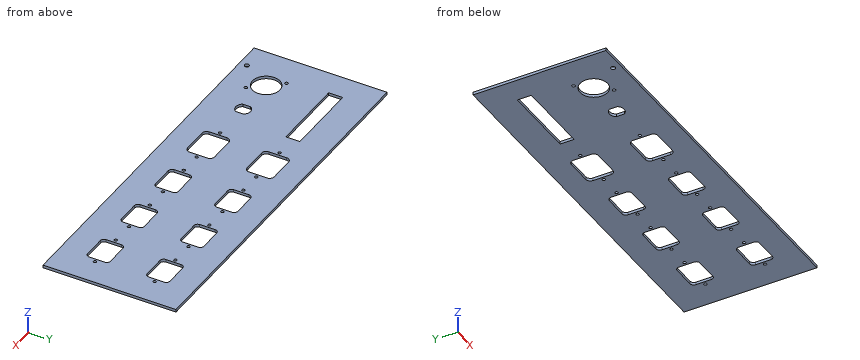
from build123d import *

# Parameters (mm, degrees)
F0_W     = 404
F0_H     = 145
F2_DEPTH = 3
F3_D     = 3.3
F3_DEPTH = 8.6
F3_TIP   = 0.9914200214
F1_R     = 1.5
F1_R_2   = 15
F1_R_3   = 1.75
F1_W     = 82
F1_H     = 15.3
F1_R_4   = 2.5
F4_DEPTH = 25


with BuildPart() as f2:
    # F0 (on Top) → F2 (new body)
    with BuildSketch(Plane.XY):
        with Locations((-14.1859020234, -7.6260944492)):
            Rectangle(F0_W, F0_H)
    extrude(amount=-F2_DEPTH)

    # F3
    with Locations(Plane.XY):
        with Locations((118.573140085, 24.8739055508), (158.573140085, 24.8739055508), (93.573140085, 24.8739055508), (53.573140085, 24.8739055508), (53.573140085, -40.1260944492), (93.573140085, -40.1260944492), (118.573140085, -40.1260944492), (158.573140085, -40.1260944492), (28.573140085, -40.1260944492), (-11.426859915, -40.1260944492), (-11.426859915, 24.8739055508), (28.573140085, 24.8739055508), (-35.926859915, 24.8739055508), (-80.926859915, 24.8739055508), (-80.926859915, -40.1260944492), (-35.926859915, -40.1260944492)):
            Hole(F3_D / 2, depth=F3_DEPTH)
            with Locations((0, 0, -(F3_DEPTH + F3_TIP / 2))):  # 118° drill point
                Cone(0, F3_D / 2, F3_TIP, mode=Mode.SUBTRACT)

    # F1 (on Top) → F4 (cut)
    with BuildSketch(Plane.XY):
        with BuildLine():
            Line((126.323140085, 12.4739055508), (150.823140085, 12.4739055508))
            ThreePointArc((150.823140085, 12.4739055508), (153.6515672098, 13.645478426), (154.823140085, 16.4739055508))
            Line((154.823140085, 16.4739055508), (154.823140085, 33.2739055508))
            ThreePointArc((154.823140085, 33.2739055508), (153.6515672098, 36.1023326755), (150.823140085, 37.2739055508))
            Line((150.823140085, 37.2739055508), (126.323140085, 37.2739055508))
            ThreePointArc((126.323140085, 37.2739055508), (123.4947129603, 36.1023326755), (122.323140085, 33.2739055508))
            Line((122.323140085, 33.2739055508), (122.323140085, 16.4739055508))
            ThreePointArc((122.323140085, 16.4739055508), (123.4947129603, 13.645478426), (126.323140085, 12.4739055508))
        make_face()
        with Locations((158.573140085, 24.8739055508)):
            Circle(F1_R)
        with Locations((118.573140085, 24.8739055508)):
            Circle(F1_R)
        with BuildLine():
            Line((-72.226859915, 10.1239055508), (-44.626859915, 10.1239055508))
            ThreePointArc((-44.626859915, 10.1239055508), (-41.091326009, 11.5883716448), (-39.626859915, 15.1239055508))
            Line((-39.626859915, 15.1239055508), (-39.626859915, 34.6239055508))
            ThreePointArc((-39.626859915, 34.6239055508), (-41.091326009, 38.1594394567), (-44.626859915, 39.6239055508))
            Line((-44.626859915, 39.6239055508), (-72.226859915, 39.6239055508))
            ThreePointArc((-72.226859915, 39.6239055508), (-75.7623938209, 38.1594394567), (-77.226859915, 34.6239055508))
            Line((-77.226859915, 34.6239055508), (-77.226859915, 15.1239055508))
            ThreePointArc((-77.226859915, 15.1239055508), (-75.7623938209, 11.5883716448), (-72.226859915, 10.1239055508))
        make_face()
        with Locations((-35.926859915, 24.8739055508)):
            Circle(F1_R)
        with Locations((-80.926859915, 24.8739055508)):
            Circle(F1_R)
        with BuildLine():
            Line((122.323140085, -31.7260944492), (122.323140085, -48.5260944492))
            ThreePointArc((122.323140085, -48.5260944492), (123.4947129603, -51.354521574), (126.323140085, -52.5260944492))
            Line((126.323140085, -52.5260944492), (150.823140085, -52.5260944492))
            ThreePointArc((150.823140085, -52.5260944492), (153.6515672098, -51.354521574), (154.823140085, -48.5260944492))
            Line((154.823140085, -48.5260944492), (154.823140085, -31.7260944492))
            ThreePointArc((154.823140085, -31.7260944492), (153.6515672098, -28.8976673245), (150.823140085, -27.7260944492))
            Line((150.823140085, -27.7260944492), (126.323140085, -27.7260944492))
            ThreePointArc((126.323140085, -27.7260944492), (123.4947129603, -28.8976673245), (122.323140085, -31.7260944492))
        make_face()
        with Locations((158.573140085, -40.1260944492)):
            Circle(F1_R)
        with Locations((118.573140085, -40.1260944492)):
            Circle(F1_R)
        with BuildLine():
            Line((57.323140085, 33.2739055508), (57.323140085, 16.4739055508))
            ThreePointArc((57.323140085, 16.4739055508), (58.4947129603, 13.645478426), (61.323140085, 12.4739055508))
            Line((61.323140085, 12.4739055508), (85.823140085, 12.4739055508))
            ThreePointArc((85.823140085, 12.4739055508), (88.6515672098, 13.645478426), (89.823140085, 16.4739055508))
            Line((89.823140085, 16.4739055508), (89.823140085, 33.2739055508))
            ThreePointArc((89.823140085, 33.2739055508), (88.6515672098, 36.1023326755), (85.823140085, 37.2739055508))
            Line((85.823140085, 37.2739055508), (61.323140085, 37.2739055508))
            ThreePointArc((61.323140085, 37.2739055508), (58.4947129603, 36.1023326755), (57.323140085, 33.2739055508))
        make_face()
        with Locations((93.573140085, 24.8739055508)):
            Circle(F1_R)
        with Locations((53.573140085, 24.8739055508)):
            Circle(F1_R)
        with BuildLine():
            Line((57.323140085, -31.7260944492), (57.323140085, -48.5260944492))
            ThreePointArc((57.323140085, -48.5260944492), (58.4947129603, -51.354521574), (61.323140085, -52.5260944492))
            Line((61.323140085, -52.5260944492), (85.823140085, -52.5260944492))
            ThreePointArc((85.823140085, -52.5260944492), (88.6515672098, -51.354521574), (89.823140085, -48.5260944492))
            Line((89.823140085, -48.5260944492), (89.823140085, -31.7260944492))
            ThreePointArc((89.823140085, -31.7260944492), (88.6515672098, -28.8976673245), (85.823140085, -27.7260944492))
            Line((85.823140085, -27.7260944492), (61.323140085, -27.7260944492))
            ThreePointArc((61.323140085, -27.7260944492), (58.4947129603, -28.8976673245), (57.323140085, -31.7260944492))
        make_face()
        with Locations((93.573140085, -40.1260944492)):
            Circle(F1_R)
        with Locations((53.573140085, -40.1260944492)):
            Circle(F1_R)
        with BuildLine():
            Line((-7.676859915, 33.2739055508), (-7.676859915, 16.4739055508))
            ThreePointArc((-7.676859915, 16.4739055508), (-6.5052870397, 13.645478426), (-3.676859915, 12.4739055508))
            Line((-3.676859915, 12.4739055508), (20.823140085, 12.4739055508))
            ThreePointArc((20.823140085, 12.4739055508), (23.6515672098, 13.645478426), (24.823140085, 16.4739055508))
            Line((24.823140085, 16.4739055508), (24.823140085, 33.2739055508))
            ThreePointArc((24.823140085, 33.2739055508), (23.6515672098, 36.1023326755), (20.823140085, 37.2739055508))
            Line((20.823140085, 37.2739055508), (-3.676859915, 37.2739055508))
            ThreePointArc((-3.676859915, 37.2739055508), (-6.5052870397, 36.1023326755), (-7.676859915, 33.2739055508))
        make_face()
        with Locations((28.573140085, 24.8739055508)):
            Circle(F1_R)
        with Locations((-11.426859915, 24.8739055508)):
            Circle(F1_R)
        with BuildLine():
            Line((-7.676859915, -31.7260944492), (-7.676859915, -48.5260944492))
            ThreePointArc((-7.676859915, -48.5260944492), (-6.5052870397, -51.354521574), (-3.676859915, -52.5260944492))
            Line((-3.676859915, -52.5260944492), (20.823140085, -52.5260944492))
            ThreePointArc((20.823140085, -52.5260944492), (23.6515672098, -51.354521574), (24.823140085, -48.5260944492))
            Line((24.823140085, -48.5260944492), (24.823140085, -31.7260944492))
            ThreePointArc((24.823140085, -31.7260944492), (23.6515672098, -28.8976673245), (20.823140085, -27.7260944492))
            Line((20.823140085, -27.7260944492), (-3.676859915, -27.7260944492))
            ThreePointArc((-3.676859915, -27.7260944492), (-6.5052870397, -28.8976673245), (-7.676859915, -31.7260944492))
        make_face()
        with Locations((28.573140085, -40.1260944492)):
            Circle(F1_R)
        with Locations((-11.426859915, -40.1260944492)):
            Circle(F1_R)
        with BuildLine():
            Line((-77.226859915, -30.3760944492), (-77.226859915, -49.8760944492))
            ThreePointArc((-77.226859915, -49.8760944492), (-75.7623938209, -53.4116283552), (-72.226859915, -54.8760944492))
            Line((-72.226859915, -54.8760944492), (-44.626859915, -54.8760944492))
            ThreePointArc((-44.626859915, -54.8760944492), (-41.091326009, -53.4116283552), (-39.626859915, -49.8760944492))
            Line((-39.626859915, -49.8760944492), (-39.626859915, -30.3760944492))
            ThreePointArc((-39.626859915, -30.3760944492), (-41.091326009, -26.8405605433), (-44.626859915, -25.3760944492))
            Line((-44.626859915, -25.3760944492), (-72.226859915, -25.3760944492))
            ThreePointArc((-72.226859915, -25.3760944492), (-75.7623938209, -26.8405605433), (-77.226859915, -30.3760944492))
        make_face()
        with Locations((-35.926859915, -40.1260944492)):
            Circle(F1_R)
        with Locations((-80.926859915, -40.1260944492)):
            Circle(F1_R)
        with Locations((-169.1859020234, -40.1260944492)):
            Circle(F1_R_2)
        with Locations((-156.6859020234, -55.1260944492)):
            Circle(F1_R_3)
        with Locations((-181.6859020234, -25.1260944492)):
            Circle(F1_R_3)
        with Locations((-147.1859020234, 24.8739055508)):
            Rectangle(F1_W, F1_H)
        with Locations((-188.1859020234, -71.9773098826)):
            Circle(F1_R_4)
        with BuildLine():
            Line((-131.9859020234, -35.8176724643), (-131.9859020234, -44.4345164341))
            ThreePointArc((-131.9859020234, -44.4345164341), (-125.1859020234, -48.1760944492), (-118.3859020234, -44.4345164341))
            Line((-118.3859020234, -44.4345164341), (-118.3859020234, -35.8176724643))
            ThreePointArc((-118.3859020234, -35.8176724643), (-125.1859020234, -32.0760944492), (-131.9859020234, -35.8176724643))
        make_face()
    extrude(amount=-F4_DEPTH, mode=Mode.SUBTRACT)


solid = f2.part
Geometry: final body of the model. Coordinates: model frame, mm. Give positions to 0.01 mm unless a question says otherwise; leave off trailing zeros. Order: outer loops, then holes, each group sorted by start corner. A loop starts at its lowest first (then second) coordinate and runs counter-clockwise, first axis right, second up. Notation, with made-up numbers: (64, 6) -> (69, 6) arc R26 cw to (69, 26) -> close; hole circle Ø1 at (-22, 36.25). An arc over 180 degrees is marked (long way). Put each result on its own line as item: value.
Q1. Section B-B, the plane z = -2.2. Count the separate pieces of the cut face and the enclosed holes in it, then the cut area to 3 significant figures.
Here are the results:
separate pieces: 1
enclosed holes: 30
area: 49,300 mm^2
Q2. Pin query (flat end, axial travel): pin 1 (4.5 mm diameter, centred on x = 118.57, y = -40.13, fed in from +Z). Return the tip coordinate at first contact, or that it passes through.
Here are the results:
pin 1: stops at z = 0
Q3. Material intervals for L1, parallel to Y at x = -171.5, z = -0.9; L2, parallel to X at y = 21, z = -2.1; L3, parallel to X at y = 17, z = -2.65, sorted ascending.
Here are the results:
L1: y = -80.13 to -54.95, -25.31 to 17.22, 32.52 to 64.87
L2: x = -216.19 to -188.19, -106.19 to -77.23, -39.63 to -7.68, 24.82 to 57.32, 89.82 to 122.32, 154.82 to 187.81
L3: x = -216.19 to -77.23, -39.63 to -7.68, 24.82 to 57.32, 89.82 to 122.32, 154.82 to 187.81
Q4. Section A-A, the plane x = 82. Return loops of the section in (y, z).
Here are the results:
outline: (-80.13, -3) -> (-52.53, -3) -> (-52.53, 0) -> (-80.13, 0) -> close; (-27.73, -3) -> (12.47, -3) -> (12.47, 0) -> (-27.73, 0) -> close; (37.27, -3) -> (64.87, -3) -> (64.87, 0) -> (37.27, 0) -> close
